Geometry: final body of the model. Coordinates: model frame, mm. A direction names the side the tool comes from. Round coordinates to 2 decimals unless told otherwise and drop trailing zeros. Write each loop counter-clockwise with the first axis right and the second up, starting at its lowest first coordinate (ties: lowest second). Pieces come first, ordered by that corner, then holes. Notation, with made-up numbers: (49.25, 3.5) - (88.25, 3.5) arc R20 cw to (88.25, 39.5) - close; hole circle Ø4 at (-30.75, 22.5). An arc over 180 degrees is marked (long way). Use a Markdown table: item, result. Add a question column.
```python
from build123d import *

# Parameters (mm, degrees)
SKETCH2_R                                       = 7.5
BOSS_EXTRUDE1_DEPTH                             = 8
CSK_FOR_M3_FLAT_HEAD_MACHINE_SCREW2_D           = 3.2
CSK_FOR_M3_FLAT_HEAD_MACHINE_SCREW2_CSINK_D     = 8.3
CSK_FOR_M3_FLAT_HEAD_MACHINE_SCREW2_CSINK_ANGLE = 90
FILLET1_R                                       = 20
V_GROOVE_CUTOUT_FLIPPED_DEPTH                   = 3.6
SKETCH49_R                                      = 2.55
CUT_EXTRUDE3_DEPTH                              = 52.922196079
CHAMFER2_SIZE                                   = 0.4
CHAMFER2_SIZE2                                  = 1.098990968
MOVE_FACE2_BY                                   = 0.5
MOVE_FACE2_2_BY                                 = 0.5
MOVE_FACE2_3_BY                                 = 0.5
MOVE_FACE2_4_BY                                 = 0.5
MOVE_FACE2_5_BY                                 = 0.5
MOVE_FACE2_6_BY                                 = 0.5
CIRPATTERN2_COUNT                               = 3
SKETCH20_R                                      = 1.375
TOOL_WING_SCREW_HOLES_DEPTH                     = 4
FILLET17_R                                      = 2
FILLET18_R                                      = 1


with BuildPart() as part:
    # Sketch2 → Boss-Extrude1 (new body)
    with BuildSketch(Plane.XY):
        Polygon((-18, 40), (18, 40), (18, -4.618802154), (32.810889132, -13.169872981), (27.810889132, -21.830127019), (-27.810889132, -21.830127019), (-32.810889132, -13.169872981), (-18, -4.618802154), align=None)
        Circle(SKETCH2_R, mode=Mode.SUBTRACT)
    extrude(amount=BOSS_EXTRUDE1_DEPTH)

    # CSK for M3 Flat Head Machine Screw2 (through all)
    with Locations(Plane.XY.offset(8)):
        with Locations((-25.980762114, -15), (0, 30), (25.980762114, -15)):
            CounterSinkHole(CSK_FOR_M3_FLAT_HEAD_MACHINE_SCREW2_D / 2, CSK_FOR_M3_FLAT_HEAD_MACHINE_SCREW2_CSINK_D / 2, counter_sink_angle=CSK_FOR_M3_FLAT_HEAD_MACHINE_SCREW2_CSINK_ANGLE)

    # Fillet1
    fillet1_edges = [part.edges().sort_by_distance(p)[0] for p in [
        (18, -4.618802154, 4),
        (-18, -4.618802154, 4),
    ]]
    fillet(fillet1_edges, radius=FILLET1_R)

    # Sketch47 → v-groove cutout flipped (cut)
    with BuildSketch(Plane(origin=(0, 0, 0), x_dir=(-1, 0, 0), z_dir=(0, 0, -1))):
        with BuildLine():
            Line((-3.464101615, 14), (-13.856406461, -4))
            ThreePointArc((-13.856406461, -4), (-13.856406461, -8), (-10.392304845, -10))
            Line((-10.392304845, -10), (10.392304845, -10))
            ThreePointArc((10.392304845, -10), (13.856406461, -8), (13.856406461, -4))
            Line((13.856406461, -4), (3.464101615, 14))
            ThreePointArc((3.464101615, 14), (0, 16), (-3.464101615, 14))
        make_face()
    extrude(amount=-V_GROOVE_CUTOUT_FLIPPED_DEPTH, mode=Mode.SUBTRACT)

    # Sketch49 → Cut-Extrude3 (cut, through all)
    with BuildSketch(Plane(origin=(0, 0, 3.6), x_dir=(-1, 0, 0), z_dir=(0, 0, -1))):
        with Locations((0, 12)):
            Circle(SKETCH49_R)
        with Locations((10.392304845, -6)):
            Circle(SKETCH49_R)
        with Locations((-10.392304845, -6)):
            Circle(SKETCH49_R)
    extrude(amount=-CUT_EXTRUDE3_DEPTH, mode=Mode.SUBTRACT)

    # Chamfer2
    chamfer2_edges = [part.edges().sort_by_distance(p)[0] for p in [
        (2.55, 12, 8),
        (-7.842304845, -6, 8),
        (12.942304845, -6, 8),
    ]]
    chamfer2_side = [part.faces().sort_by_distance(p)[0] for p in [
        (17.098380214, 23.464101615, 8),
    ]]
    chamfer(chamfer2_edges, length=CHAMFER2_SIZE, length2=CHAMFER2_SIZE2, reference=chamfer2_side[0])

    # Move Face2: a curved face moved inward by 0.5
    add(Solid.thicken(part.faces().sort_by_distance((-13.856406461, -8, 1.8))[0], -MOVE_FACE2_BY), mode=Mode.SUBTRACT)

    # Move Face2 2: a face moved inward by 0.5
    extrude(part.faces().sort_by_distance((0, -10, 1.8))[0], amount=MOVE_FACE2_2_BY, dir=(0, -1, 0), mode=Mode.SUBTRACT)

    # Move Face2 3: a curved face moved inward by 0.5
    add(Solid.thicken(part.faces().sort_by_distance((13.856406461, -8, 1.8))[0], -MOVE_FACE2_3_BY), mode=Mode.SUBTRACT)

    # Move Face2 4: a face moved inward by 0.5
    extrude(part.faces().sort_by_distance((8.660254038, 5, 1.8))[0], amount=MOVE_FACE2_4_BY, dir=(0.866025404, 0.5, 0), mode=Mode.SUBTRACT)

    # Move Face2 5: a curved face moved inward by 0.5
    add(Solid.thicken(part.faces().sort_by_distance((0, 16, 1.8))[0], -MOVE_FACE2_5_BY), mode=Mode.SUBTRACT)

    # Move Face2 6: a face moved inward by 0.5
    extrude(part.faces().sort_by_distance((-8.660254038, 5, 1.8))[0], amount=MOVE_FACE2_6_BY, dir=(-0.866025404, 0.5, 0), mode=Mode.SUBTRACT)

    # Sketch46 → tool ball cutout (revolve, cut)
    with BuildSketch(Plane(origin=(0, 30, 0), x_dir=(1, 0, 0), z_dir=(0, 1, 0))):
        with BuildLine():
            Line((0, 4.3), (0, -3.7))
            ThreePointArc((0, -3.7), (-4, 0.3), (0, 4.3))
        make_face()
    tool_ball_cutout = revolve(axis=Axis((0, 30, 0), (0, 0, -1)), mode=Mode.SUBTRACT)

    # CirPattern2: tool ball cutout ×3 about axis
    cirpattern2_axis = Axis((0, 0, 0), (0, 0, 1))
    for i in range(1, CIRPATTERN2_COUNT):
        add(tool_ball_cutout.rotate(cirpattern2_axis, i * 360 / CIRPATTERN2_COUNT), mode=Mode.SUBTRACT)

    # Sketch20 → Tool Wing Screw Holes (cut)
    with BuildSketch(Plane(origin=(18, 0, 0), x_dir=(0, 0, -1), z_dir=(1, 0, 0))):
        with Locations(Location((-4, 19, 0), (0, 0, 90))):
            Circle(SKETCH20_R)
        with Locations(Location((-4, 32.5, 0), (0, 0, 90))):
            Circle(SKETCH20_R)
    tool_wing_screw_holes = extrude(amount=-TOOL_WING_SCREW_HOLES_DEPTH, mode=Mode.SUBTRACT)

    # Mirror2: Tool Wing Screw Holes across plane
    add(tool_wing_screw_holes.mirror(Plane(origin=(0, 0, 0), x_dir=(0, 0, 1), z_dir=(1, 0, 0))), mode=Mode.SUBTRACT)

    # Fillet17
    fillet17_edges = [part.edges().sort_by_distance(p)[0] for p in [
        (32.810889132, -13.169872981, 4),
        (27.810889132, -21.830127019, 4),
        (-27.810889132, -21.830127019, 4),
        (-32.810889132, -13.169872981, 4),
    ]]
    fillet(fillet17_edges, radius=FILLET17_R)

    # Fillet18
    fillet18_edges = [part.edges().sort_by_distance(p)[0] for p in [
        (-18, 40, 4),
        (18, 40, 4),
    ]]
    fillet(fillet18_edges, radius=FILLET18_R)


solid = part.part
```
1) Material intervals for L1, parallel to Y at x = 0, z = 4.9; L2, parallel to X at y = -15, z = 1; L3, parallel to Z at x = 16.05, y = 19 (3 decimals), sorted ascending. Write a range as from..to.
2) Section A-A, the plane y = 30. Return the cut outline in (x, z).
3) Section C-C, the plane y = 19. Return the cut outline in (x, z) (3 decimals).
4) Section D-D, the plane x = -0.5. State how many separate pieces and enclosed holes the cut face has, then the cut area to 3 significant figures.
5) Section B-B, the plane y = -6. Return the cut outline in (x, z).
6) Pin query (flat end, axial travel): P1, Ø2, axis at y = 32.5, z = 4, coming from the +X side; P2, Ø3.5, axis at x = 0, y = 30, coming from the -Z side; P3, Ø3, axis at y = 19, z = 4, coming from the +X side. Return the tip coordinate at first contact, or that it passes through.
7) Draft query along Y for faces 6 (the flat face through (8, 10, 0)), 7 (the cylindrical face through (27.16, -13.92, 4.39)), 8 (the flat face through (-30.076, -17.908, 3.944)). Return one class per face: released by +Y, released by -Y, zero draft, split by the parting line, or undercut.
8) Set-up query: faces 1 (the flat face through (-9.17, 5.12, 1.77)), 2 (the flat face through (-14, 19, 4)), 3 (the cylindrical face through (12.94, -5.89, 5.23)), 4 (the flat face through (-18, 23, 4)), 5 (the flat face through (14, 32, 4)). Return all of +Z, -Z, +X, -X, +Y, -Y with unobstructed straight access to the full face (end or side cutting, diameter ignored); none if empty.
Output values:
| question | item | result |
|---|---|---|
| 1 | L1 | y = -21.83..-7.5, 7.5..9.45, 14.55..28.4, 31.6..40 |
| 1 | L2 | x = -31.75..-29.76, -22.2..22.2, 29.76..31.75 |
| 1 | L3 | z = 0..2.625, 5.375..8 |
| 2 | outline | (-18, 0) - (-3.99, 0) arc R4 cw to (-1.6, 3.37) - (-1.6, 5.45) - (-4.15, 8) - (-18, 8) - close; (1.6, 3.37) arc R4 cw to (3.99, 0) - (18, 0) - (18, 8) - (4.15, 8) - (1.6, 5.45) - close |
| 3 | outline | (-18, 0) - (18, 0) - (18, 2.625) - (14, 2.625) - (14, 5.375) - (18, 5.375) - (18, 8) - (-18, 8) - (-18, 5.375) - (-14, 5.375) - (-14, 2.625) - (-18, 2.625) - close |
| 4 | separate pieces | 4 |
| 4 | enclosed holes | 0 |
| 4 | area | 267 mm^2 |
| 5 | outline | (-22.74, 0) - (-14.89, 0) - (-14.89, 3.6) - (-12.94, 3.6) - (-12.94, 6.9) - (-13.34, 8) - (-22.74, 8) - close; (-7.84, 3.6) - (-4.5, 3.6) - (-4.5, 8) - (-7.44, 8) - (-7.84, 6.9) - close; (4.5, 3.6) - (7.84, 3.6) - (7.84, 6.9) - (7.44, 8) - (4.5, 8) - close; (12.94, 3.6) - (14.89, 3.6) - (14.89, 0) - (22.74, 0) - (22.74, 8) - (13.34, 8) - (12.94, 6.9) - close |
| 6 | P1 | stops at x = 14 |
| 6 | P2 | stops at z = 3.3 |
| 6 | P3 | stops at x = 18 |
| 7 | face 6 | zero draft |
| 7 | face 7 | undercut |
| 7 | face 8 | released by -Y |
| 8 | face 1 | -Z |
| 8 | face 2 | -X |
| 8 | face 3 | +Z, -Z |
| 8 | face 4 | +Z, -Z, -X, +Y |
| 8 | face 5 | +X |
